from build123d import *

# Parameters (mm, degrees)
BOX006_W     = 23
BOX006_H     = 7
BOX006_DEPTH = 10
BOX005_W     = 69
BOX005_H     = 7
BOX005_DEPTH = 10
BOX004_W     = 24
BOX004_H     = 7
BOX004_DEPTH = 10
BOX003_W     = 2
BOX003_H     = 4
BOX003_DEPTH = 10
BOX002_W     = 2
BOX002_H     = 4
BOX002_DEPTH = 10
BOX001_W     = 148
BOX001_H     = 14
BOX001_DEPTH = 2
BOX_W        = 150
BOX_H        = 16
BOX_DEPTH    = 3
BOX011_W     = 69
BOX011_H     = 7
BOX011_DEPTH = 10
BOX012_W     = 23
BOX012_H     = 7
BOX012_DEPTH = 10
BOX010_W     = 24
BOX010_H     = 7
BOX010_DEPTH = 10
BOX008_W     = 1
BOX008_H     = 3
BOX008_DEPTH = 1
BOX007_W     = 1
BOX007_H     = 3
BOX007_DEPTH = 1
BOX009_W     = 150
BOX009_H     = 16
BOX009_DEPTH = 0.5


with BuildPart() as cube006:
    # Box006 → Box006 (new body)
    with BuildSketch(Plane(origin=(122, 3.5, -3), x_dir=(1, 0, 0), z_dir=(0, 0, 1))):
        with Locations((11.5, 3.5)):
            Rectangle(BOX006_W, BOX006_H)
    extrude(amount=BOX006_DEPTH)


with BuildPart() as cube005:
    # Box005 → Box005 (new body)
    with BuildSketch(Plane(origin=(41, 3.5, -3), x_dir=(1, 0, 0), z_dir=(0, 0, 1))):
        with Locations((34.5, 3.5)):
            Rectangle(BOX005_W, BOX005_H)
    extrude(amount=BOX005_DEPTH)


with BuildPart() as cube004:
    # Box004 → Box004 (new body)
    with BuildSketch(Plane(origin=(6, 3.5, -3), x_dir=(1, 0, 0), z_dir=(0, 0, 1))):
        with Locations((12, 3.5)):
            Rectangle(BOX004_W, BOX004_H)
    extrude(amount=BOX004_DEPTH)


with BuildPart() as cube003:
    # Box003 → Box003 (new body)
    with BuildSketch(Plane(origin=(115, 0.8, -5), x_dir=(1, 0, 0), z_dir=(0, 0, 1))):
        with Locations((1, 2)):
            Rectangle(BOX003_W, BOX003_H)
    extrude(amount=BOX003_DEPTH)


with BuildPart() as cube002:
    # Box002 → Box002 (new body)
    with BuildSketch(Plane(origin=(34, 0.7, -5), x_dir=(1, 0, 0), z_dir=(0, 0, 1))):
        with Locations((1, 2)):
            Rectangle(BOX002_W, BOX002_H)
    extrude(amount=BOX002_DEPTH)


with BuildPart() as cube001:
    # Box001 → Box001 (new body)
    with BuildSketch(Plane(origin=(2, 0, 1), x_dir=(1, 0, 0), z_dir=(0, 0, 1))):
        with Locations((74, 7)):
            Rectangle(BOX001_W, BOX001_H)
    extrude(amount=BOX001_DEPTH)


with BuildPart() as cut005:
    # Box → Box (new body)
    with BuildSketch(Plane.XY):
        with Locations((75, 8)):
            Rectangle(BOX_W, BOX_H)
    extrude(amount=BOX_DEPTH)

    # Cut: cut Cube001
    add(cube001.part, mode=Mode.SUBTRACT)

    # Cut001: cut Cube002
    add(cube002.part, mode=Mode.SUBTRACT)

    # Cut002: cut Cube003
    add(cube003.part, mode=Mode.SUBTRACT)

    # Cut003: cut Cube004
    add(cube004.part, mode=Mode.SUBTRACT)

    # Cut004: cut Cube005
    add(cube005.part, mode=Mode.SUBTRACT)

    # Cut005: cut Cube006
    add(cube006.part, mode=Mode.SUBTRACT)


with BuildPart() as cube011:
    # Box011 → Box011 (new body)
    with BuildSketch(Plane(origin=(41, 3.5, -3), x_dir=(1, 0, 0), z_dir=(0, 0, 1))):
        with Locations((34.5, 3.5)):
            Rectangle(BOX011_W, BOX011_H)
    extrude(amount=BOX011_DEPTH)


with BuildPart() as cube012:
    # Box012 → Box012 (new body)
    with BuildSketch(Plane(origin=(122, 3.5, -3), x_dir=(1, 0, 0), z_dir=(0, 0, 1))):
        with Locations((11.5, 3.5)):
            Rectangle(BOX012_W, BOX012_H)
    extrude(amount=BOX012_DEPTH)


with BuildPart() as cube010:
    # Box010 → Box010 (new body)
    with BuildSketch(Plane(origin=(6, 3.5, -3), x_dir=(1, 0, 0), z_dir=(0, 0, 1))):
        with Locations((12, 3.5)):
            Rectangle(BOX010_W, BOX010_H)
    extrude(amount=BOX010_DEPTH)


with BuildPart() as cube008:
    # Box008 → Box008 (new body)
    with BuildSketch(Plane(origin=(115.5, 1.3, 0), x_dir=(1, 0, 0), z_dir=(0, 0, 1))):
        with Locations((0.5, 1.5)):
            Rectangle(BOX008_W, BOX008_H)
    extrude(amount=BOX008_DEPTH)


with BuildPart() as cube007:
    # Box007 → Box007 (new body)
    with BuildSketch(Plane(origin=(34.5, 1.2, 0), x_dir=(1, 0, 0), z_dir=(0, 0, 1))):
        with Locations((0.5, 1.5)):
            Rectangle(BOX007_W, BOX007_H)
    extrude(amount=BOX007_DEPTH)


with BuildPart() as fusion001:
    # Box009 → Box009 (new body)
    with BuildSketch(Plane.XY.offset(-0.5)):
        with Locations((75, 8)):
            Rectangle(BOX009_W, BOX009_H)
    extrude(amount=BOX009_DEPTH)

    # Fusion: union Cube008, Cube007
    add(cube008.part)
    add(cube007.part)

    # Cut006: cut Cube010
    add(cube010.part, mode=Mode.SUBTRACT)

    # Cut007: cut Cube012
    add(cube012.part, mode=Mode.SUBTRACT)

    # Cut008: cut Cube011
    add(cube011.part, mode=Mode.SUBTRACT)

    # Fusion001: union Cut005
    add(cut005.part)


solid = fusion001.part
Could you check a few things on this model? Use its own coordinates, in mm. A direction names the side the tool comes from. Coordinates: 2 decimals unless noted, no trailing zeros. Order: outer loops, then holes, each group sorted by start corner. A loop starts at its lowest first (then second) coordinate and runs counter-clockwise, first axis right, second up. Notation, with made-up numbers: (-26.5, 3.5) - (-21.5, 3.5) arc R21 ccw to (-21.5, 15.5) - close; hole circle Ø9 at (-2, 15.5). An arc over 180 degrees is marked (long way). Answer in a Markdown table with one row per item. Add a question column.
(1) I need wall thicknesses on L1, parallel to X at y = 5.75, z = 0.3; L2, parallel to X at y = 3, z = 0.3; L3, parallel to Y at x = 105, z = 0.4. Which ranges of each line are inside material? Lowest first, please.
(2) If we section it at B-B, the plane y = 7.5: Please give me the cut outline in (x, z).
(3) If we mould it in two halves opening along X, with no side actions, what happens to faces 1 (the face through (0, 8, 1)), 2 (the face through (150, 8, 0)), 3 (the face through (74, 0, 0))? For each: released by +X, released by -X, zero draft, split by the parting line, or undercut.
(4) Will this pin go through, and if not, where does the flat tip stop? pin 1 (1 mm diameter, centred on x = 35, y = 3.5, fed in from +Z).
(5) If we section it at C-C, the plane z = 2: Please give me the cut outline in (x, y).
(6) If we section it at A-A, the plane x = 20: Please give me the cut outline in (y, z), then the cut area to 3 significant figures.
(7) On a 3-axis mill with a long thin cutter (end or side, diameter ignored), from which of +Z, -Z, +X, -X, +Y, -Y can I reach the whole of each face in a straight line? I mean faces 4 (the face through (75, 12, 1)), 5 (the face through (75, 15, 3)). Say none if no direction works.
(8) If we section it at D-D, the plane x = 112.5: Please give me the cut outline in (y, z), then the cut area to 3 significant figures.
Results are:
| question | item | result |
|---|---|---|
| 1 | L1 | x = 0 to 6, 30 to 41, 110 to 122, 145 to 150 |
| 1 | L2 | x = 0 to 34, 34.5 to 35.5, 36 to 115, 115.5 to 116.5, 117 to 150 |
| 1 | L3 | y = 0 to 3.5, 10.5 to 16 |
| 2 | outline | (0, -0.5) - (6, -0.5) - (6, 1) - (2, 1) - (2, 3) - (0, 3) - close; (30, -0.5) - (41, -0.5) - (41, 1) - (30, 1) - close; (110, -0.5) - (122, -0.5) - (122, 1) - (110, 1) - close; (145, -0.5) - (150, -0.5) - (150, 1) - (145, 1) - close |
| 3 | face 1 | released by -X |
| 3 | face 2 | released by +X |
| 3 | face 3 | zero draft |
| 4 | pin 1 | stops at z = 1 |
| 5 | outline | (0, 0) - (2, 0) - (2, 14) - (150, 14) - (150, 16) - (0, 16) - close |
| 6 | outline | (0, -0.5) - (3.5, -0.5) - (3.5, 1) - (0, 1) - close; (10.5, -0.5) - (16, -0.5) - (16, 3) - (14, 3) - (14, 1) - (10.5, 1) - close |
| 6 | area | 17.5 mm2 |
| 7 | face 4 | +Z, +X, -Y |
| 7 | face 5 | +Z, +X, -X, +Y, -Y |
| 8 | outline | (0, -0.5) - (16, -0.5) - (16, 3) - (14, 3) - (14, 1) - (0, 1) - close |
| 8 | area | 28.0 mm2 |
